from build123d import *

# Parameters (mm, degrees)
REVOLVE_1_ANGLE                    = 180
EXTRUDE_START                      = -20
EXTRUDE_1_DEPTH                    = 20
EXTRUDE_2_REACH                    = 90.73
SKETCH_3_W                         = 28
SKETCH_3_H                         = 65
CUT_EXTRUDE_1_DEPTH                = 3
CUT_EXTRUDE_1_DEPTH_BACK           = 3
SKETCH_4_R                         = 4
CUT_EXTRUDE_2_REACH                = 90.006
SKETCH_5_R                         = 2.1
EXTRUDE_3_DEPTH                    = 18
CUT_EXTRUDE_3_REACH                = 92.692
SKETCH_7_R                         = 2.1
CUT_EXTRUDE_4_REACH                = 83.394
SKETCH_8_R                         = 1.1
SKETCH_9_R                         = 1.9
CUT_EXTRUDE_5_DEPTH                = 0.5
SKETCH_10_R                        = 1.9
CUT_EXTRUDE_6_DEPTH                = 1.2
CUT_EXTRUDE_6_DRAFT                = -45
PATTERN_CIRCULAR_1_COUNT           = 2
PATTERN_CIRCULAR_1_ANGLE           = 60
PATTERN_CIRCULAR_1_COPY_1_SKETCH_R = 1.9
PATTERN_CIRCULAR_1_COPY_1_DEPTH    = 1.2
PATTERN_CIRCULAR_1_COPY_1_DRAFT    = -45
HOLE_WIZARD_M31_AT_2_COUNT         = 2
HOLE_WIZARD_M31_AT_2_PITCH         = 15
PATTERN_CIRCULAR_2_COUNT           = 2
PATTERN_CIRCULAR_2_ANGLE           = 90
FILLET_1_R                         = 0.4
FILLET_2_R                         = 4


# Read off the part's stored shape, not the designer's step: Бобышка-Вытянуть1
with BuildPart() as part:
    # Эскиз1 → Повернуть1 (revolve)
    with BuildSketch(Plane(origin=(0, 0, 0), x_dir=(1, 0, 0), z_dir=(0, 1, 0))):
        Polygon((-11, 85), (-14, 85), (-14, 20), (-18, 20), (-18, 0), (-12.5, 0), (-12.5, 10), (-6, 10), (-6, 11), (-7.5, 11), (-7.5, 14), (-11, 14), align=None)
    revolve(axis=Axis((0, 0, 0), (0, 0, 1)), revolution_arc=REVOLVE_1_ANGLE)

    # Бобышка-Вытянуть1 outline → Бобышка-Вытянуть1 (add)
    with BuildSketch(Plane.XY.offset(EXTRUDE_START)):
        with BuildLine():
            Line((-18, -18), (0, -18))
            ThreePointArc((0, -18), (-12.727922061, -12.727922061), (-18, 0))
            Line((-18, 0), (-18, -18))
        make_face()
        with BuildLine():
            Line((18, -18), (18, 0))
            ThreePointArc((18, 0), (12.727922061, -12.727922061), (0, -18))
            Line((0, -18), (18, -18))
        make_face()
    extrude(amount=EXTRUDE_1_DEPTH)

    # Эскиз3 → Бобышка-Вытянуть2 (add, up to next)
    with BuildSketch(Plane(origin=(0, -18, 0), x_dir=(1, 0, 0), z_dir=(0, 1, 0)), mode=Mode.PRIVATE) as extrude_2_sk1:
        with Locations((0, 52.5)):
            Rectangle(SKETCH_3_W, SKETCH_3_H)
    extrude_2_tool1 = extrude(extrude_2_sk1.sketch, amount=EXTRUDE_2_REACH, mode=Mode.PRIVATE) - part.part
    add(extrude_2_tool1.solids().sort_by_distance((0, -18, -52.5))[0])

    # Эскиз4 → Вырез-Вытянуть1 (cut, two sides: drawn at the far end of the back side and taken through both)
    with BuildSketch(Plane(origin=(0, -11, 0), x_dir=(1, 0, 0), z_dir=(0, 1, 0)).offset(-CUT_EXTRUDE_1_DEPTH_BACK)):
        with Locations(Location((0, 70, 0), (0, 0, 90))):
            Circle(SKETCH_4_R)
    extrude(amount=CUT_EXTRUDE_1_DEPTH + CUT_EXTRUDE_1_DEPTH_BACK, mode=Mode.SUBTRACT)

    # Эскиз5 → Вырез-Вытянуть2 (cut, up to next)
    with BuildSketch(Plane(origin=(0, -14, 0), x_dir=(1, 0, 0), z_dir=(0, 1, 0)), mode=Mode.PRIVATE) as cut_extrude_2_sk1:
        with Locations(Location((0, 70, 0), (0, 0, 270))):
            Circle(SKETCH_5_R)
    cut_extrude_2_tool1 = extrude(cut_extrude_2_sk1.sketch, amount=-CUT_EXTRUDE_2_REACH, mode=Mode.PRIVATE) & part.part
    add(cut_extrude_2_tool1.solids().sort_by_distance((0, -14, -70))[0], mode=Mode.SUBTRACT)

    # Эскиз6 → Бобышка-Вытянуть3 (add)
    with BuildSketch(Plane(origin=(0, -18, 0), x_dir=(1, 0, 0), z_dir=(0, 1, 0))):
        with BuildLine():
            Line((14, 20), (22, 20))
            ThreePointArc((22, 20), (26, 24), (22, 28))
            Line((22, 28), (14, 28))
            Line((14, 28), (14, 20))
        make_face()
    extrude_3 = extrude(amount=EXTRUDE_3_DEPTH)

    # Эскиз7 → Вырез-Вытянуть3 (cut, up to next)
    with BuildSketch(Plane(origin=(0, 0, 0), x_dir=(1, 0, 0), z_dir=(0, 1, 0)), mode=Mode.PRIVATE) as cut_extrude_3_sk1:
        with Locations(Location((22, 24, 0), (0, 0, 180))):
            Circle(SKETCH_7_R)
    cut_extrude_3_tool1 = extrude(cut_extrude_3_sk1.sketch, amount=-CUT_EXTRUDE_3_REACH, mode=Mode.PRIVATE) & part.part
    cut_extrude_3 = cut_extrude_3_tool1.solids().sort_by_distance((22, 0, -24))[0]
    add(cut_extrude_3, mode=Mode.SUBTRACT)

    # Зеркальное отражение1: Бобышка-Вытянуть3, Вырез-Вытянуть3 across plane
    add(extrude_3.mirror(Plane(origin=(0, 0, 0), x_dir=(0, 0, 1), z_dir=(1, 0, 0))))
    add(cut_extrude_3.mirror(Plane(origin=(0, 0, 0), x_dir=(0, 0, 1), z_dir=(1, 0, 0))), mode=Mode.SUBTRACT)

    # Эскиз8 → Вырез-Вытянуть4 (cut, up to next)
    with BuildSketch(Plane.XY.offset(-10), mode=Mode.PRIVATE) as cut_extrude_4_sk1:
        with Locations((-4.75, -8.227241336)):
            Circle(SKETCH_8_R)
    cut_extrude_4_tool1 = extrude(cut_extrude_4_sk1.sketch, amount=-CUT_EXTRUDE_4_REACH, mode=Mode.PRIVATE) & part.part
    cut_extrude_4 = cut_extrude_4_tool1.solids().sort_by_distance((-4.75, -8.227241, -10))[0]
    add(cut_extrude_4, mode=Mode.SUBTRACT)

    # Эскиз9 → Вырез-Вытянуть5 (cut)
    with BuildSketch(Plane.XY.offset(-10)):
        with Locations((-4.75, -8.227241336)):
            Circle(SKETCH_9_R)
    cut_extrude_5 = extrude(amount=-CUT_EXTRUDE_5_DEPTH, mode=Mode.SUBTRACT)


with BuildPart() as cut_extrude_6_tool:
    # Эскиз10 → Вырез-Вытянуть6 (with draft: the straight prism first)
    with BuildSketch(Plane.XY.offset(-10.5)):
        with Locations((-4.75, -8.227241336)):
            Circle(SKETCH_10_R)
    extrude(amount=-CUT_EXTRUDE_6_DEPTH)
    # Вырез-Вытянуть6: the draft: its side faces are tilted about the plane it starts from
    cut_extrude_6_sides = [cut_extrude_6_tool.faces().sort_by_distance(p)[0] for p in [
        (-6.65, -8.227241336, -11.1),
    ]]
    draft(cut_extrude_6_sides, Plane.XY.offset(-10.5), CUT_EXTRUDE_6_DRAFT)


with BuildPart() as part_1:
    add(part.part)

    # Вырез-Вытянуть6: cut by cut_extrude_6_tool
    add(cut_extrude_6_tool.part, mode=Mode.SUBTRACT)

    # Круговой массив1: Вырез-Вытянуть4, Вырез-Вытянуть5 ×2 about axis
    pattern_circular_1_axis = Axis((0, 0, 0), (0, 0, 1))
    add([cut_extrude_4.rotate(pattern_circular_1_axis, i * PATTERN_CIRCULAR_1_ANGLE / (PATTERN_CIRCULAR_1_COUNT - 1)) for i in range(1, PATTERN_CIRCULAR_1_COUNT)], mode=Mode.SUBTRACT)
    add([cut_extrude_5.rotate(pattern_circular_1_axis, i * PATTERN_CIRCULAR_1_ANGLE / (PATTERN_CIRCULAR_1_COUNT - 1)) for i in range(1, PATTERN_CIRCULAR_1_COUNT)], mode=Mode.SUBTRACT)


with BuildPart() as pattern_circular_1_copy_1_tool:
    # Круговой массив1 copy 1 sketch → Круговой массив1 copy 1 (with draft: the straight prism first)
    with BuildSketch(Plane(origin=(0, 0, -10.5), x_dir=(0.4999999999999978, 0.8660254037844399, 0), z_dir=(0, 0, 1))):
        with Locations((-4.75, -8.227241336)):
            Circle(PATTERN_CIRCULAR_1_COPY_1_SKETCH_R)
    extrude(amount=-PATTERN_CIRCULAR_1_COPY_1_DEPTH)
    # Круговой массив1 copy 1: the draft: its side faces are tilted about the plane it starts from
    pattern_circular_1_copy_1_sides = [pattern_circular_1_copy_1_tool.faces().sort_by_distance(p)[0] for p in [
        (3.8, -9.872689603, -11.1),
    ]]
    draft(pattern_circular_1_copy_1_sides, Plane(origin=(0, 0, -10.5), x_dir=(0.4999999999999978, 0.8660254037844399, 0), z_dir=(0, 0, 1)), PATTERN_CIRCULAR_1_COPY_1_DRAFT)


with BuildPart() as part_2:
    add(part_1.part)

    # Круговой массив1 copy 1: cut by pattern_circular_1_copy_1_tool
    add(pattern_circular_1_copy_1_tool.part, mode=Mode.SUBTRACT)

    # Эскиз11 → Сверление под метчик M31 (revolve, cut)
    with BuildSketch(Plane(origin=(10.606601718, -10.606601718, 0), x_dir=(0, -1, 0), z_dir=(1, 0, 0))):
        Polygon((0, 0), (0, 15.751075774), (1.25, 15), (1.25, 0), align=None)
    hole_wizard_m31 = revolve(axis=Axis((10.606601718, -10.606601718, 6.35), (0, 0, -1)), mode=Mode.SUBTRACT)

    # Сверление под метчик M31 at 2: Сверление под метчик M31 ×2
    with Locations(*[Vector(-0.7071067811865464, 0.7071067811865487, 0) * (i * HOLE_WIZARD_M31_AT_2_PITCH) for i in range(1, HOLE_WIZARD_M31_AT_2_COUNT)]):
        add(hole_wizard_m31, mode=Mode.SUBTRACT)

    # Круговой массив2: Сверление под метчик M31 ×2 about axis
    pattern_circular_2_axis = Axis((0, 0, 0), (0, 0, -1))
    for i in range(1, PATTERN_CIRCULAR_2_COUNT):
        add(hole_wizard_m31.rotate(pattern_circular_2_axis, i * PATTERN_CIRCULAR_2_ANGLE / (PATTERN_CIRCULAR_2_COUNT - 1)), mode=Mode.SUBTRACT)

    # Круговой массив2 copy 1 sketch → Круговой массив2 copy 1 (revolve, cut)
    with BuildSketch(Plane(origin=(0, 0, 0), x_dir=(-1, 0, 0), z_dir=(0, -1, 0))):
        Polygon((0, 0), (0, 15.751075774), (1.25, 15), (1.25, 0), align=None)
    revolve(axis=Axis((0, 0, 6.35), (0, 0, -1)), mode=Mode.SUBTRACT)

    # Скругление1
    fillet_1_edges = [part_2.edges().sort_by_distance(p)[0] for p in [
        (18, -9, -20),
        (-18, -9, -20),
        (14, -9, -28),
        (-14, -9, -28),
    ]]
    fillet(fillet_1_edges, radius=FILLET_1_R)

    # Скругление2
    fillet_2_edges = [part_2.edges().sort_by_distance(p)[0] for p in [
        (-14, -9, -85),
        (14, -9, -85),
    ]]
    fillet(fillet_2_edges, radius=FILLET_2_R)


solid = part_2.part
Here's how the part is built. I have some questions about the finished solid (model axes, mm). A direction names the side the tool comes from. Round coordinates to 2 decimals unless told otherwise and drop trailing zeros. Order: outer loops, then holes, each group sorted by start corner. A loop starts at its lowest first (then second) coordinate and runs counter-clockwise, first axis right, second up. Notation, with made-up numbers: (70.5, 80.5) -> (100.5, 80.5) arc R36 cw to (100.5, 119.5) -> close; hole circle Ø1 at (-21.5, -25). An arc over 180 degrees is marked (long way). Return JSON: item names as keys, results as strings.
Q1. For pin 1 Ø2.5 at (x, y) = (4.75, -8.23) entering from +Z; pin 2 Ø8 at (y, z) = (-2.5, -38.5) entering from +X; pin 3 Ø6.5 at (x, z) = (-1.5, -69) entering from +Y, each with a flat end and sliding along its axis, tell me the tip position at first contact or that it passes through.
Filled sheet:
{"pin 1": "stops at z = -11.15", "pin 2": "stops at x = 14", "pin 3": "stops at y = -9.92"}
Q2. If we section it at A-A on z = -70: List the corners of the cut face in (x, y) for me, plus the area to 3 significant figures.
Filled sheet:
{"outline": "(-14, -18) -> (-2.1, -18) -> (-2.1, -14) -> (-4, -14) -> (-4, -10.25) arc R11 cw to (-11, 0) -> (-14, 0) -> close; (2.1, -18) -> (14, -18) -> (14, 0) -> (11, 0) arc R11 cw to (4, -10.25) -> (4, -14) -> (2.1, -14) -> close", "area": "271 mm^2"}
Q3. If we section it at D-D on z = -5.5: List the corners of the cut face in (x, y) for me, plus the area to 3 significant figures.
Filled sheet:
{"outline": "(-18, -18) -> (18, -18) -> (18, 0) -> (12.5, 0) arc R12.5 cw to (-12.5, 0) -> (-18, 0) -> close; hole circle Ø2.5 at (-10.61, -10.61); hole circle Ø2.5 at (10.61, -10.61)", "area": "393 mm^2"}
Q4. I need wall thicknesses on line 1 along Z through (x, y) = (22, -9.25); line 2 along Z through (x, y) = (15, -16.75); line 3 along X through (y, z) = (-3.5, -27.5). Which ranges of each line are inside material? Lowest first, please. Write a range as from..to.
Filled sheet:
{"line 1": "z = -28..-26.1, -21.9..-20", "line 2": "z = -28..0", "line 3": "x = -23.94..-10.43, 10.43..23.94"}
Q5. If we section it at B-B on x = 0: List the corners of the cut face in (y, z) for me, plus the area to 3 significant figures.
Filled sheet:
{"outline": "(-18, -85) -> (-11, -85) -> (-11, -74) -> (-14, -74) -> (-14, -72.1) -> (-18, -72.1) -> close; (-18, -67.9) -> (-14, -67.9) -> (-14, -66) -> (-11, -66) -> (-11, -14) -> (-7.5, -14) -> (-7.5, -11) -> (-6, -11) -> (-6, -10) -> (-12.5, -10) -> (-12.5, 0) -> (-18, 0) -> close", "area": "555 mm^2"}
Q6. Which directions (+Z, -Z, +X, -X, +Y, -Y) give clear straight access to the entire face, cutting with the end or side of a thin tool? Please do faces 4 (the cylindrical face through (6.65, -8.31, -10.25)), 5 (the flat face through (0.2, -6.3, -10)), 6 (the flat face through (-14, -9, -54)), 7 (the flat face through (2, -14, -72)), 8 (the flat face through (-20, -9, -20)).
Filled sheet:
{"face 4": "+Z", "face 5": "+Z, +Y", "face 6": "-Z, -X, +Y, -Y", "face 7": "+Y", "face 8": "+Z, -X, +Y, -Y"}
Q7. If we mould it in two halves opening along Z, with no side actions, what happens to faces 1 (the conical face through (-10.814, -10.541, -15.621)), 2 (the flat face through (13.7, 0, -30.1)), 3 (the cylindrical face through (-20.87, -8.87, -22.23))? For each: released by +Z, released by -Z, zero draft, split by the parting line, or undercut.
Filled sheet:
{"face 1": "released by +Z", "face 2": "zero draft", "face 3": "undercut"}
Q8. If we section it at C-C on z = -24: List the corners of the cut face in (x, y) for me.
Filled sheet:
{"outline": "(-26, -18) -> (-24.1, -18) -> (-24.1, 0) -> (-26, 0) -> close; (-19.9, -18) -> (19.9, -18) -> (19.9, 0) -> (11, 0) arc R11 cw to (-11, 0) -> (-19.9, 0) -> close; (24.1, -18) -> (26, -18) -> (26, 0) -> (24.1, 0) -> close"}
